Input: part model. Units: mm. Frame: model coordinates. A direction names the side the tool comes from. Round coordinates to 2 decimals unless told otherwise and drop trailing zeros. Loops run counter-clockwise (first coordinate to the right, second up) from the corner with the lowest first, then second, coordinate; pieces in that order, holes last. Notation, with made-up numbers: M -18,-3.75 L -8,-3.75 A27 cw -8,31.25 Z; hole C -16,1.25 d10. An arc over 180 degrees is marked long. Put each result on its own line as item: value. Start each with the question number.
1) Section C-C on x = -7.14. Output: boundary loops of the cut face in (y, z).
2) Section D-D on z = 3.5. Output: boundary loops of the cut face in (x, y).
3) Reachability of faces 1 (the face through (0, 38, 4)), 2 (the face through (-10, 54, -1)), 3 (the face through (-10, 24, 1)), 4 (the face through (-16.8, 38, 4)) from +Z, -Z, +X, -X, +Y, -Y: full face, straight path, thin tool, end or side. Return the list, or none.
4) Pin query (flat end, axial travel): pin 1 (2 mm diameter, centred on x = -7.14, y = 6.6, fed in from +Z); pin 2 (5 mm diameter, centred on x = -8, y = 55, fed in from +Z); pin 3 (3.5 mm diameter, centred on x = -9, z = 3, fed in from -Y). Return the tip coordinate at first contact, or that it passes through.
5) Section B-B on x = -2.75. Output: boundary loops of the cut face in (y, z), plus the area to 3 significant figures.
6) Draft query along X for faces 5 (the face through (-19, 12, 1)), 6 (the face through (-15.88, 15.04, -0.54)), 7 (the face through (-9, 41, 4)). Return one class per face: +X half, -X half, draft (parallel to the pull), parting line (faces both ways), or undercut.
7) Line query: probe 1 along Z at (x, y) = (-8.5, 38); probe 2 along Y at (x, z) = (-2.75, 0.25); probe 3 along Y at (x, z) = (-9.5, -0.45). Output: solid intervals per line, ascending.
8) Section A-A on y = 6.6. Output: boundary loops of the cut face in (x, z), plus the area to 4 significant figures.
from build123d import *

# Parameters (mm, degrees)
F0_W     = 4.1414871812
F0_H     = 3
F0_W_2   = 25
F0_H_2   = 35.3582080007
F0_R     = 3
F0_W_3   = 3.0508699417
F0_W_4   = 6.3956826925
F0_W_5   = 5.4119601846
F0_W_6   = 19
F0_H_3   = 13.8665742949
F0_R_2   = 0.65
F1_DEPTH = 3
F2_DEPTH = 2
F6_DEPTH = 15.5
F7_R     = 3
F8_DEPTH = 2
F9_DEPTH = 1.3


with BuildPart() as f1:
    # F0 (on Top) → F1 (new body)
    with BuildSketch(Plane.XY):
        with Locations((-2.0707435906, -1.5)):
            Rectangle(F0_W, F0_H)
        with Locations((-9.5, 44.6791040003)):
            Rectangle(F0_W_2, F0_H_2)
        with Locations((-9.5, 54.3582080007)):
            Circle(F0_R, mode=Mode.SUBTRACT)
        with Locations((-17.4745650291, -1.5)):
            Rectangle(F0_W_3, F0_H)
        with Locations((-7.3393285275, -1.5)):
            Rectangle(F0_W_4, F0_H)
        Polygon((0, 10.1334257051), (0, 0), (0, -3), (3, -3), (3, 27), (-22, 27), (-22, -3), (-19, -3), (-19, 0), (-19, 10.1334257051), (-19, 24), (0, 24), align=None)
        with Locations((-13.243149966, -1.5)):
            Rectangle(F0_W_5, F0_H)
        with Locations((-9.5, 17.0667128526)):
            Rectangle(F0_W_6, F0_H_3)
        with Locations((-15.8, 16)):
            Circle(F0_R_2, mode=Mode.SUBTRACT)
        with Locations((-15.4, 14.6)):
            Circle(F0_R_2, mode=Mode.SUBTRACT)
        with Locations((-14.9, 17.8)):
            Circle(F0_R_2, mode=Mode.SUBTRACT)
        Polygon((-4.1414871812, 0), (0, 0), (0, 10.1334257051), (-19, 10.1334257051), (-19, 0), (-15.9491300583, 0), (-10.5371698737, 0), align=None)
        with Locations((-7.14, 6.6)):
            Circle(F0_R_2, mode=Mode.SUBTRACT)
        with Locations((-5.1, 8.7)):
            Circle(F0_R_2, mode=Mode.SUBTRACT)
    extrude(amount=-F1_DEPTH)

    # F0 (on Top) → F2 (join)
    with BuildSketch(Plane.XY):
        with Locations((-9.5, 17.0667128526)):
            Rectangle(F0_W_6, F0_H_3)
        with Locations((-15.8, 16)):
            Circle(F0_R_2, mode=Mode.SUBTRACT)
        with Locations((-15.4, 14.6)):
            Circle(F0_R_2, mode=Mode.SUBTRACT)
        with Locations((-14.9, 17.8)):
            Circle(F0_R_2, mode=Mode.SUBTRACT)
        Polygon((-4.1414871812, 0), (0, 0), (0, 10.1334257051), (-19, 10.1334257051), (-19, 0), (-15.9491300583, 0), (-10.5371698737, 0), align=None)
        with Locations((-7.14, 6.6)):
            Circle(F0_R_2, mode=Mode.SUBTRACT)
        with Locations((-5.1, 8.7)):
            Circle(F0_R_2, mode=Mode.SUBTRACT)
    extrude(amount=F2_DEPTH)

    # F5 (on offset) → F6 (join)
    with BuildSketch(Plane(origin=(-16.8, 0, 0), x_dir=(0, -1, 0), z_dir=(-1, 0, 0))):
        with BuildLine():
            ThreePointArc((-35, 7), (-38, 10), (-41, 7))
            Line((-41, 7), (-39.75, 7))
            ThreePointArc((-39.75, 7), (-38, 8.75), (-36.25, 7))
            Line((-36.25, 7), (-35, 7))
        make_face()
        with BuildLine():
            Line((-41, 7), (-41, 0))
            Line((-41, 0), (-35, 0))
            Line((-35, 0), (-35, 7))
            Line((-35, 7), (-36.25, 7))
            ThreePointArc((-36.25, 7), (-38, 5.25), (-39.75, 7))
            Line((-39.75, 7), (-41, 7))
        make_face()
    extrude(amount=-F6_DEPTH)

    # F7 (on face) → F8 (join)
    with BuildSketch(Plane(origin=(0, 0, -3), x_dir=(1, 0, 0), z_dir=(0, 0, -1))):
        with Locations((-9.5, -54.3582080007)):
            Circle(F7_R)
    extrude(amount=-F8_DEPTH)

    # F9 (add): a face of the model
    f9_faces = [f1.faces().sort_by_distance(p)[0] for p in [
        (-1.3, 38, 4.2267630358),
    ]]
    extrude(f9_faces, amount=F9_DEPTH)


solid = f1.part
Geometry results:
1. outline: M -3,-3 L 5.95,-3 L 5.95,2 L 0,2 L 0,0 L -3,0 Z; M 7.25,-3 L 62.36,-3 L 62.36,0 L 56.21,0 L 56.21,-1 L 52.51,-1 L 52.51,0 L 41,0 L 41,7 A3 ccw 35,7 L 35,0 L 24,0 L 24,2 L 7.25,2 Z; hole C 38,7 d3.5
2. outline: M -16.8,35 L 0,35 L 0,41 L -16.8,41 Z
3. face 1: +Z, +X, +Y, -Y
3. face 2: +Z
3. face 3: +Z, +X, -X
3. face 4: +Z, -X, +Y
4. pin 1: stops at z = 2
4. pin 2: stops at z = 0
4. pin 3: stops at y = 0
5. outline: M -3,-3 L 62.36,-3 L 62.36,0 L 41,0 L 41,7 A3 ccw 35,7 L 35,0 L 24,0 L 24,2 L 0,2 L 0,0 L -3,0 Z; hole C 38,7 d3.5
5. area: 291 mm²
6. face 5: -X half
6. face 6: undercut
6. face 7: draft
7. probe 1: z = -3 to 5.25, 8.75 to 10
7. probe 2: y = 0 to 24, 35 to 41
7. probe 3: y = -3 to 51.36, 57.36 to 62.36
8. outline: M -22,-3 L -7.79,-3 L -7.79,2 L -19,2 L -19,0 L -22,0 Z; M -6.49,-3 L 3,-3 L 3,0 L 0,0 L 0,2 L -6.49,2 Z
8. area: 106.5 mm²
